Check sheet for the modelled part. Datum: model origin and axes. Units: mm. Face numbers are marked on the shaded views. A direction names the side the tool comes from. Coordinates: 2 decimals unless noted, no trailing zeros. Write each loop counter-clockwise with the first axis right and the second up, starting at its lowest first coordinate (ties: lowest second). Pieces come first, ordered by that corner, then holes. Notation, with made-up numbers: (0.5, -27.5) -> (43.5, -27.5) arc R9 cw to (43.5, -15.5) -> close; hole circle Ø3 at (5.5, -13.75). An arc over 180 degrees is marked (long way). Put each result on its own line as item: value.
```python
from build123d import *

# Parameters (mm, degrees)
SKETCH1_W           = 51.5
SKETCH1_H           = 20
BOSS_EXTRUDE1_DEPTH = 3.5
SKETCH2_W           = 12
SKETCH2_H           = 18
BOSS_EXTRUDE2_DEPTH = 3.5
FILLET1_R           = 1
FILLET2_R           = 1
SKETCH3_W           = 12
SKETCH3_H           = 18
BOSS_EXTRUDE3_DEPTH = 3.5
FILLET3_R           = 1
FILLET4_R           = 1
FILLET5_R           = 1
FILLET6_R           = 1
FILLET7_R           = 1
FILLET8_R           = 1
FILLET9_R           = 1
FILLET10_R          = 1
FILLET11_R          = 1
FILLET12_R          = 1
SKETCH4_W           = 12
SKETCH4_H           = 1.95
BOSS_EXTRUDE4_DEPTH = 7
SKETCH5_W           = 12
SKETCH5_H           = 1.95
BOSS_EXTRUDE5_DEPTH = 7
FILLET13_R          = 1
FILLET14_R          = 1
FILLET15_R          = 1
FILLET16_R          = 1
FILLET17_R          = 1
SKETCH8_W           = 16.25
SKETCH8_H           = 25.726511914
BOSS_EXTRUDE6_DEPTH = 11.42
FILLET21_R          = 2
FILLET22_R          = 2
FILLET23_R          = 2
SKETCH9_R           = 0.745983734
CUT_EXTRUDE1_DEPTH  = 10
SKETCH10_R          = 0.75
CUT_EXTRUDE2_DEPTH  = 10
SKETCH11_R          = 1.41875541
CUT_EXTRUDE3_DEPTH  = 10
SKETCH12_R          = 1.401780947
CUT_EXTRUDE4_DEPTH  = 10


with BuildPart() as part:
    # Sketch1 → Boss-Extrude1 (new body)
    with BuildSketch(Plane.XY):
        Rectangle(SKETCH1_W, SKETCH1_H)
    extrude(amount=BOSS_EXTRUDE1_DEPTH)

    # Sketch2 → Boss-Extrude2 (add)
    with BuildSketch(Plane(origin=(0, 10, 0), x_dir=(1, 0, 0), z_dir=(0, 1, 0))):
        with Locations((11.75, -10.75)):
            Rectangle(SKETCH2_W, SKETCH2_H)
    extrude(amount=BOSS_EXTRUDE2_DEPTH)

    # Fillet1
    fillet1_edges = [part.edges().sort_by_distance(p)[0] for p in [
        (11.75, 10, 1.75),
    ]]
    fillet(fillet1_edges, radius=FILLET1_R)

    # Fillet2
    fillet2_edges = [part.edges().sort_by_distance(p)[0] for p in [
        (11.75, 10, 3.5),
    ]]
    fillet(fillet2_edges, radius=FILLET2_R)

    # Sketch3 → Boss-Extrude3 (add)
    with BuildSketch(Plane(origin=(0, -10, 0), x_dir=(-1, 0, 0), z_dir=(0, -1, 0))):
        with Locations((-11.75, -10.75)):
            Rectangle(SKETCH3_W, SKETCH3_H)
    extrude(amount=BOSS_EXTRUDE3_DEPTH)

    # Fillet3
    fillet3_edges = [part.edges().sort_by_distance(p)[0] for p in [
        (11.75, -10, 1.75),
    ]]
    fillet(fillet3_edges, radius=FILLET3_R)

    # Fillet4
    fillet4_edges = [part.edges().sort_by_distance(p)[0] for p in [
        (11.75, -10, 3.5),
    ]]
    fillet(fillet4_edges, radius=FILLET4_R)

    # Fillet5
    fillet5_edges = [part.edges().sort_by_distance(p)[0] for p in [
        (17.75, 10, 2.125),
    ]]
    fillet(fillet5_edges, radius=FILLET5_R)

    # Fillet6
    fillet6_edges = [part.edges().sort_by_distance(p)[0] for p in [
        (5.75, 10, 2.125),
    ]]
    fillet(fillet6_edges, radius=FILLET6_R)

    # Fillet7
    fillet7_edges = [part.edges().sort_by_distance(p)[0] for p in [
        (17.75, 10, 3.5),
    ]]
    fillet(fillet7_edges, radius=FILLET7_R)

    # Fillet8
    fillet8_edges = [part.edges().sort_by_distance(p)[0] for p in [
        (5.75, 10, 3.5),
    ]]
    fillet(fillet8_edges, radius=FILLET8_R)

    # Fillet9
    fillet9_edges = [part.edges().sort_by_distance(p)[0] for p in [
        (5.75, -10, 2.125),
    ]]
    fillet(fillet9_edges, radius=FILLET9_R)

    # Fillet10
    fillet10_edges = [part.edges().sort_by_distance(p)[0] for p in [
        (5.75, -10, 3.5),
    ]]
    fillet(fillet10_edges, radius=FILLET10_R)

    # Fillet11
    fillet11_edges = [part.edges().sort_by_distance(p)[0] for p in [
        (17.75, -10, 2.125),
    ]]
    fillet(fillet11_edges, radius=FILLET11_R)

    # Fillet12
    fillet12_edges = [part.edges().sort_by_distance(p)[0] for p in [
        (17.75, -10, 3.5),
    ]]
    fillet(fillet12_edges, radius=FILLET12_R)

    # Sketch4 → Boss-Extrude4 (add)
    with BuildSketch(Plane(origin=(0, -10, 0), x_dir=(1, 0, 0), z_dir=(0, 1, 0))):
        with Locations((11.75, -18.775)):
            Rectangle(SKETCH4_W, SKETCH4_H)
    extrude(amount=BOSS_EXTRUDE4_DEPTH)

    # Sketch5 → Boss-Extrude5 (add)
    with BuildSketch(Plane(origin=(0, 10, 0), x_dir=(-1, 0, 0), z_dir=(0, -1, 0))):
        with Locations((-11.75, -18.775)):
            Rectangle(SKETCH5_W, SKETCH5_H)
    extrude(amount=BOSS_EXTRUDE5_DEPTH)

    # Fillet13
    fillet13_edges = [part.edges().sort_by_distance(p)[0] for p in [
        (11.75, 10, 17.8),
    ]]
    fillet(fillet13_edges, radius=FILLET13_R)

    # Fillet14
    fillet14_edges = [part.edges().sort_by_distance(p)[0] for p in [
        (11.75, 13.5, 19.75),
    ]]
    fillet(fillet14_edges, radius=FILLET14_R)

    # Fillet15
    fillet15_edges = [part.edges().sort_by_distance(p)[0] for p in [
        (11.75, 13.5, 1.75),
    ]]
    fillet(fillet15_edges, radius=FILLET15_R)

    # Fillet16
    fillet16_edges = [part.edges().sort_by_distance(p)[0] for p in [
        (11.75, -13.5, 19.75),
    ]]
    fillet(fillet16_edges, radius=FILLET16_R)

    # Fillet17
    fillet17_edges = [part.edges().sort_by_distance(p)[0] for p in [
        (11.75, -10, 17.8),
    ]]
    fillet(fillet17_edges, radius=FILLET17_R)

    # Sketch8 → Boss-Extrude6 (add)
    with BuildSketch(Plane(origin=(0, 0, 0), x_dir=(-1, 0, 0), z_dir=(0, 0, -1))):
        with Locations((17.625, -2.863255957)):
            Rectangle(SKETCH8_W, SKETCH8_H)
    extrude(amount=BOSS_EXTRUDE6_DEPTH)

    # Fillet21
    fillet21_edges = [part.edges().sort_by_distance(p)[0] for p in [
        (-9.5, 0, 0),
    ]]
    fillet(fillet21_edges, radius=FILLET21_R)

    # Fillet22
    fillet22_edges = [part.edges().sort_by_distance(p)[0] for p in [
        (-17.625, -10, 0),
    ]]
    fillet(fillet22_edges, radius=FILLET22_R)

    # Fillet23
    fillet23_edges = [part.edges().sort_by_distance(p)[0] for p in [
        (-9.5, -10, 0),
    ]]
    fillet(fillet23_edges, radius=FILLET23_R - 0.0001)  # a hair under: the kernel refuses the full size

    # Sketch9 → Cut-Extrude1 (cut)
    with BuildSketch(Plane(origin=(0, 0, 0), x_dir=(-1, 0, 0), z_dir=(0, 0, -1))):
        with Locations((-23.742674676, -0.005014859)):
            Circle(SKETCH9_R)
    extrude(amount=-CUT_EXTRUDE1_DEPTH, mode=Mode.SUBTRACT)

    # Sketch10 → Cut-Extrude2 (cut)
    with BuildSketch(Plane(origin=(0, 0, 0), x_dir=(-1, 0, 0), z_dir=(0, 0, -1))):
        with Locations((-1.39, 0)):
            Circle(SKETCH10_R)
    extrude(amount=-CUT_EXTRUDE2_DEPTH, mode=Mode.SUBTRACT)

    # Sketch11 → Cut-Extrude3 (cut)
    with BuildSketch(Plane(origin=(0, 0, -11.42), x_dir=(-1, 0, 0), z_dir=(0, 0, -1))):
        with Locations((16.518366767, 3.994492079)):
            Circle(SKETCH11_R)
    extrude(amount=-CUT_EXTRUDE3_DEPTH, mode=Mode.SUBTRACT)

    # Sketch12 → Cut-Extrude4 (cut)
    with BuildSketch(Plane(origin=(0, 0, -11.42), x_dir=(-1, 0, 0), z_dir=(0, 0, -1))):
        with Locations((16.50448956, -9.000225668)):
            Circle(SKETCH12_R)
    extrude(amount=-CUT_EXTRUDE4_DEPTH, mode=Mode.SUBTRACT)


solid = part.part
```
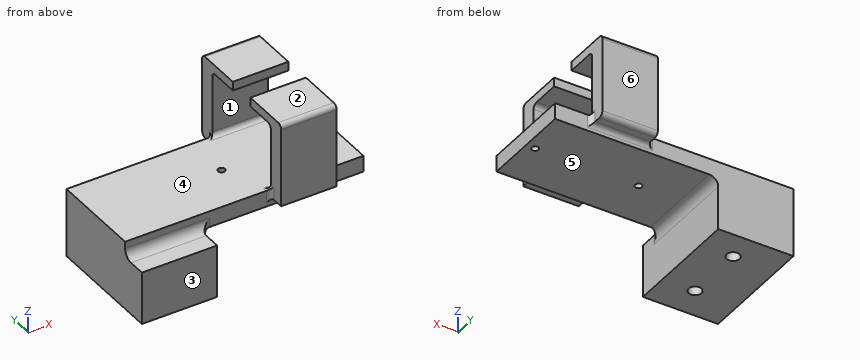
Q1. Cross-section at C-C (z = 6). Record the cut outline in (x, y).
Recorded:
outline: (5.75, -13.5) -> (17.75, -13.5) -> (17.75, -10) -> (5.75, -10) -> close; (5.75, 10) -> (17.75, 10) -> (17.75, 13.5) -> (5.75, 13.5) -> close
Q2. Mould release check, pull along Y, two halves, no side actions. Record for the marked faces 3, 4, 5 and 6: released by +Y, released by -Y, zero draft, split by the parting line, or undercut.
Recorded:
face 3: released by -Y
face 4: undercut
face 5: zero draft
face 6: released by +Y
Q3. Tool access check on the marked faces 1 and 2. Record the directions out of +Z, -Z, +X, -X, +Y, -Y that give a thin tool (end or side, any length) a straight path to the whole face; none if there is none.
Recorded:
face 1: +X, -X
face 2: +Z, +X, -X, +Y, -Y
Q4. Cross-section at D-D (x = 10). Record the cut outline in (y, z), plus the area to 3 significant figures.
Recorded:
outline: (-13.5, 1.75) -> (-11, 1.75) arc R1 cw to (-10, 0.75) -> (-10, 0) -> (10, 0) -> (10, 0.75) arc R1 cw to (11, 1.75) -> (12.5, 1.75) arc R1 ccw to (13.5, 2.75) -> (13.5, 18.75) arc R1 ccw to (12.5, 19.75) -> (3, 19.75) -> (3, 17.8) -> (9, 17.8) arc R1 cw to (10, 16.8) -> (10, 4.5) arc R1 cw to (9, 3.5) -> (-9, 3.5) arc R1 cw to (-10, 4.5) -> (-10, 16.8) arc R1 cw to (-9, 17.8) -> (-3, 17.8) -> (-3, 19.75) -> (-12.5, 19.75) arc R1 ccw to (-13.5, 18.75) -> close
area: 224 mm2
Q5. Cross-section at B-B (x = 1.39). Record the cut outline in (y, z), plus the area to 4 significant figures.
Recorded:
outline: (-10, 0) -> (-0.75, 0) -> (-0.75, 3.5) -> (-10, 3.5) -> close; (0.75, 0) -> (10, 0) -> (10, 3.5) -> (0.75, 3.5) -> close
area: 64.75 mm2
Q6. Cross-section at A-A (y = -7). Record the cut outline in (x, z), plus the area to 3 significant figures.
Recorded:
outline: (-25.75, -11.42) -> (-9.5, -11.42) -> (-9.5, -2) arc R2 cw to (-7.5, 0) -> (25.75, 0) -> (25.75, 3.5) -> (-25.75, 3.5) -> close; (5.75, 17.8) -> (17.75, 17.8) -> (17.75, 19.75) -> (5.75, 19.75) -> close
area: 390 mm2
Q7. Material ranges on line 1 along Y through (x, z) = (11.5, 9); line 2 along Z through (x, y) = (7.5, 5); line 3 along Z through (x, y) = (15, 1.75), recorded low to high.
Recorded:
line 1: y = -13.5 to -10, 10 to 13.5
line 2: z = 0 to 3.5, 17.8 to 19.75
line 3: z = 0 to 3.5
Q8. Depth check by flat-ended pin: P1, Ø3, axis at x = 4, z = 12.5, coming from the -Y side; P2, Ø1.7, axis at x = 23.74, y = -0.01, coming from the -Z side; P3, Ø5.5, axis at y = -5, z = -7.5, coming from the +X side; P4, Ø1.4, axis at x = -16.5, y = -8.5, coming from the -Z side. Enter the tip coordinate at first touch or a pass-through.
Recorded:
P1: passes through
P2: stops at z = 0
P3: stops at x = -9.5
P4: stops at z = -1.42
